Part model, mm, in its own coordinate system. A direction names the side the tool comes from. Round coordinates to 2 decimals unless told otherwise and drop trailing zeros. Order: outer loops, then holes, each group sorted by start corner. A loop starts at its lowest first (then second) coordinate and runs counter-clockwise, first axis right, second up. Notation, with made-up numbers: (80.5, -30) -> (109.5, -30) arc R32 cw to (109.5, 6) -> close; hole circle Ø6 at (68.5, 11.5). An arc over 180 degrees is marked (long way). Use CSV: the item, a comma, the result in double quotes.
Autodesk Inventor part; units mm, degrees
ref_plane "YZ Plane" through (0, 0, 0) normal (1, 0, 0) x (0, 1, 0)
ref_plane "XZ Plane" through (0, 0, 0) normal (0, 1, 0) x (-1, 0, 0)
ref_plane "XY Plane" through (0, 0, 0) normal (0, 0, 1) x (1, 0, 0)
sketch "Sketch1" plane through (0, 0, 0) normal (0, 0, 1) x (1, 0, 0)
  line L0 (0, 0) -> (0, 15)
  line L1 (0, 15) -> (5.5, 15)
  line L2 (5.5, 15) -> (5.5, 14)
  line L3 (5.5, 14) -> (4.25, 14)
  line L4 (4.25, 14) -> (4.25, 7)
  line L5 (4.25, 7) -> (5.1, 7)
  line L6 (5.5, 6.6) -> (5.5, 0)
  line L7 (5.5, 0) -> (0, 0)
  line L8 (-2.5, 11.781) -> (-2.5, 3.2351)
  line L9 (5.5, 6.6) -> (5.1, 7)
  point P0 (5.5, 7)
  dimension "d0" = 5.5
  dimension "d1" = 7
  dimension "d2" = 7
  dimension "d4" = 2.5
  dimension "d6" = 15
  dimension "d7" = 4.25
  dimension "d8" = 0.4
  dimension "d9" = 0.4
revolve "Revolution2" add sketch "Sketch1" angle 360 about axis through (-2.5, 11.781, 0) along (0, -1, 0)
properties part number "gt2_20_pulley"
(1) Which spindle directions (+Z, -Z, +X, -X, +Y, -Y) get a long thin tool onto all of the face, cutting with end or side? Do faces 4 (the face through (-4.23, 3.25, -7.81)), 5 (the face through (-7.857, 10.451, -4.107)). Say none if no direction does.
Reply:
face 4,"+Y, -Y"
face 5,"none"
(2) Probe probe 1 along Z at (x, y) = (-2.5, 6.5); probe 2 along X at (y, z) = (3.25, 2.25); probe 3 along X at (y, z) = (12.75, -1.5). List the from-to ranges inside material, lowest first. Write a range as [from, to].
Reply:
probe 1,"[-8, -2.5], [2.5, 8]"
probe 2,"[-10.18, -3.59], [-1.41, 5.18]"
probe 3,"[-9.08, -4.5], [-0.5, 4.08]"
(3) Drop flat-ended pins along their axis: P1, Ø2, axis at x = -7, y = 11, coming from the -Z side; P2, Ø1.5, axis at y = 3, z = -3.5, coming from the -X side; P3, Ø1.5, axis at y = 7.5, z = 4.5, coming from the -X side. Give the stop position or say it passes through.
Reply:
P1,"z = -5.77"
P2,"x = -10.01"
P3,"x = -9.06"
(4) Pull direction Z, two halves, no side cores. Call faces 1 (the face through (-0.115, 7.605, -0.751)), 2 (the face through (-4.23, 14.49, -7.81)), 3 (the face through (-4.4, 0, 1.9)): released by +Z, released by -Z, zero draft, split by the parting line, or undercut.
Reply:
face 1,"undercut"
face 2,"split by the parting line"
face 3,"zero draft"
(5) Cut at B-B, the plane x = -2.5. Give the cut face in (y, z), then the cut area to 3 significant figures.
Reply:
outline,"(0, -8) -> (6.6, -8) -> (7, -7.6) -> (7, -6.75) -> (14, -6.75) -> (14, -8) -> (15, -8) -> (15, -2.5) -> (0, -2.5) -> close; (0, 2.5) -> (15, 2.5) -> (15, 8) -> (14, 8) -> (14, 6.75) -> (7, 6.75) -> (7, 7.6) -> (6.6, 8) -> (0, 8) -> close"
area,"147 mm2"
(6) Cut at C-C, the plane y = 6.25. Give the cut face in (x, z).
Reply:
outline,"circle Ø16 at (-2.5, 0); hole circle Ø5 at (-2.5, 0)"
(7) Cut at A-A, the plane z = 0. Give the cut face in (x, y), then the cut area to 3 significant figures.
Reply:
outline,"(-10.5, 0) -> (-5, 0) -> (-5, 15) -> (-10.5, 15) -> (-10.5, 14) -> (-9.25, 14) -> (-9.25, 7) -> (-10.1, 7) -> (-10.5, 6.6) -> close; (0, 0) -> (5.5, 0) -> (5.5, 6.6) -> (5.1, 7) -> (4.25, 7) -> (4.25, 14) -> (5.5, 14) -> (5.5, 15) -> (0, 15) -> close"
area,"147 mm2"
